Input: part model. Units: mm. Frame: model coordinates. A direction names the side the tool comes from. Give positions to 0.01 mm unless a question says otherwise; leave off trailing zeros. Order: outer loops, then holes, each group sorted by start corner. A loop starts at its lowest first (then second) coordinate and runs counter-clockwise, first axis right, second up. Notation, with made-up numbers: (84.5, -35) -> (88.5, -35) arc R5 ccw to (88.5, -27) -> close; hole circle Ø9 at (68.25, -2.5). An arc over 180 degrees is marked (long way). Use a Markdown table: item, result. Add a question column.
Autodesk Inventor part; units mm, degrees
ref_plane "YZ Plane" through (0, 0, 0) normal (1, 0, 0) x (0, 1, 0)
ref_plane "XZ Plane" through (0, 0, 0) normal (0, 1, 0) x (-1, 0, 0)
ref_plane "XY Plane" through (0, 0, 0) normal (0, 0, 1) x (1, 0, 0)
sketch "Skizze1" plane through (0, 0, 0) normal (0, 0, 1) x (1, 0, 0)
  circle A0 centre (0, 0) radius 100
  circle A1 centre (0, 0) radius 95.1
  circle A2 centre (0, 0) radius 89.6
  circle A3 centre (0, 0) radius 25
  dimension "d0" = 200
  dimension "d1" = 4.9
  dimension "d2" = 5.5
  dimension "d7" = 50
extrude "Extrusion1" add sketch "Skizze1" along normal blind 4.9 contours A0 | A1 | A2
extrude "Extrusion2" add sketch "Skizze1" against normal blind 59 contours A1
equation "\"d0\" = kg_diameter"
equation "\"d1\" = kg_thickness"
equation "\"d7\" = ht_diameter"
equation "\"d3\" = kg_thickness"
equation "\"kg_diameter\" = 200"
equation "\"kg_thickness\" = 4.9"
equation "\"ht_diameter\" = 50"
equation "\"ht_thickness\" = 1.9"
equation "\"case_thickness\" = 18"
equation "\"gap_fit\" = 0.1"
equation "\"gap_slide\" = 0.2"
equation "\"gap_air\" = 1"
equation "\"bore_diameter\" = 73"
equation "\"tape_thickness\" = 3"
equation "\"mdf_thickness\" = 6"
equation "\"tape_width\" = 15"
equation "\"inner_thickness\" = 15"
equation "\"inner_depth\" = 255"
properties part number "Zyklon_Deckel"
Q1. First-contact query: pin 1 (10 mm diameter, centred on y = -76, z = -49, fed in from -X); pin 2 (10 mm diameter, centred on x = 28, y = -66, fed in from -Z); pin 3 (1 mm diameter, centred on x = -51.5, z = -39, fed in from +Y). Flat tips, straight axial feed; report the tip coordinate or a pass-through.
Q2. Ray query, line 1 (Y direction, x = 0, z = 2.2); line 2 (Y direction, x = 0, z = -44.5); line 3 (X direction, y = 49, z = -14). Return the intervals inside material, ascending.
Q3. Section query C-C (z = -54.5). Return loops of the section in (x, y), plus the area to 3 significant figures.
Q4. Draft query along Y for faces 3 (the cylindrical face through (23.846, -7.509, 2.416)), 4 (the cylindrical face through (-75.468, -57.867, -29.087)), 5 (the flat face through (-29, 85, -59)). Return one class per face: +Y half, -Y half, draft (parallel to the pull), parting line (faces both ways), or undercut.
Q5. Section query A-A (y = 0). Return loops of the section in (x, z).
Q6. Access query for faces 1 (the flat face through (21, -21, 4.9)), 2 (the cylindrical face through (-89.513, 3.94, -29.087)). Directions: +Z, -Z, +X, -X, +Y, -Y. A direction counts if a zero-diameter tool reaches every point of the face in a straight line with its end or side. Return the directions, or none.
Q7. Section query D-D (y = -39.5). Return loops of the section in (x, z), plus the area to 3 significant figures.
Solution:
| question | item | result |
|---|---|---|
| 1 | pin 1 | stops at x = -63.27 |
| 1 | pin 2 | stops at z = 0 |
| 1 | pin 3 | stops at y = 80.27 |
| 2 | line 1 | y = -100 to -25, 25 to 100 |
| 2 | line 2 | y = -95.1 to -89.6, 89.6 to 95.1 |
| 2 | line 3 | x = -81.5 to -75.01, 75.01 to 81.5 |
| 3 | outline | circle Ø190.2 at (0, 0); hole circle Ø179.2 at (0, 0) |
| 3 | area | 3,190 mm² |
| 4 | face 3 | undercut |
| 4 | face 4 | parting line |
| 4 | face 5 | draft |
| 5 | outline | (-100, 0) -> (-95.1, 0) -> (-95.1, -59) -> (-89.6, -59) -> (-89.6, 0) -> (-25, 0) -> (-25, 4.9) -> (-100, 4.9) -> close; (25, 0) -> (89.6, 0) -> (89.6, -59) -> (95.1, -59) -> (95.1, 0) -> (100, 0) -> (100, 4.9) -> (25, 4.9) -> close |
| 6 | face 1 | +Z, +X, -X, +Y, -Y |
| 6 | face 2 | -Z |
| 7 | outline | (-91.87, 0) -> (-86.51, 0) -> (-86.51, -59) -> (-80.42, -59) -> (-80.42, 0) -> (80.42, 0) -> (80.42, -59) -> (86.51, -59) -> (86.51, 0) -> (91.87, 0) -> (91.87, 4.9) -> (-91.87, 4.9) -> close |
| 7 | area | 1,620 mm² |
